Part print with two shaded views. Sizes in mm from the minimum x, y, z corner. Give positions to 0.01 mm unless a question says otherwise; leave off trailing zeros. Loops run counter-clockwise (first coordinate to the right, second up) from the corner with the lowest first, then second, coordinate; pieces in that order, holes last. Notation, with made-up numbers: M -23,70 L 12,70 A37 cw 12,109 Z; hole C 33,-2 d3. An arc over 180 degrees is marked long. Answer as a JSON object with one key per item and string values. Group by question number.
1. Mould opens along Z. For the marked faces 1 and 2 say: released by +Z, released by -Z, zero draft, split by the parting line, or undercut.
2. Slice it at C-C (z = 2.5). List the corners of the cut face in (x, y).
3. Drop flat-ended pins along their axis: pin 1 Ø1 at (y, z) = (42, 21.5) entering from -X; pin 2 Ø6 at (x, z) = (11, 7.5) entering from -Y; pin 3 Ø10 at (x, y) = (18, 37) entering from -Z. Give the stop position or say it passes through.
4. Slice it at A-A (z = 12.5). List the corners of the cut face in (x, y) (1 decimal).
5. Slice it at D-D (y = 24.13). List the corners of the cut face in (x, z).
6. Drill centre lines: line 1 along Z through (x, y) = (24.13, 44.25); line 2 along Y through (x, z) = (27, 20.5) (1 decimal); line 3 along Y through (x, z) = (21, 6). Where is each one in solid material? Low to high. Write a range as [from, to].
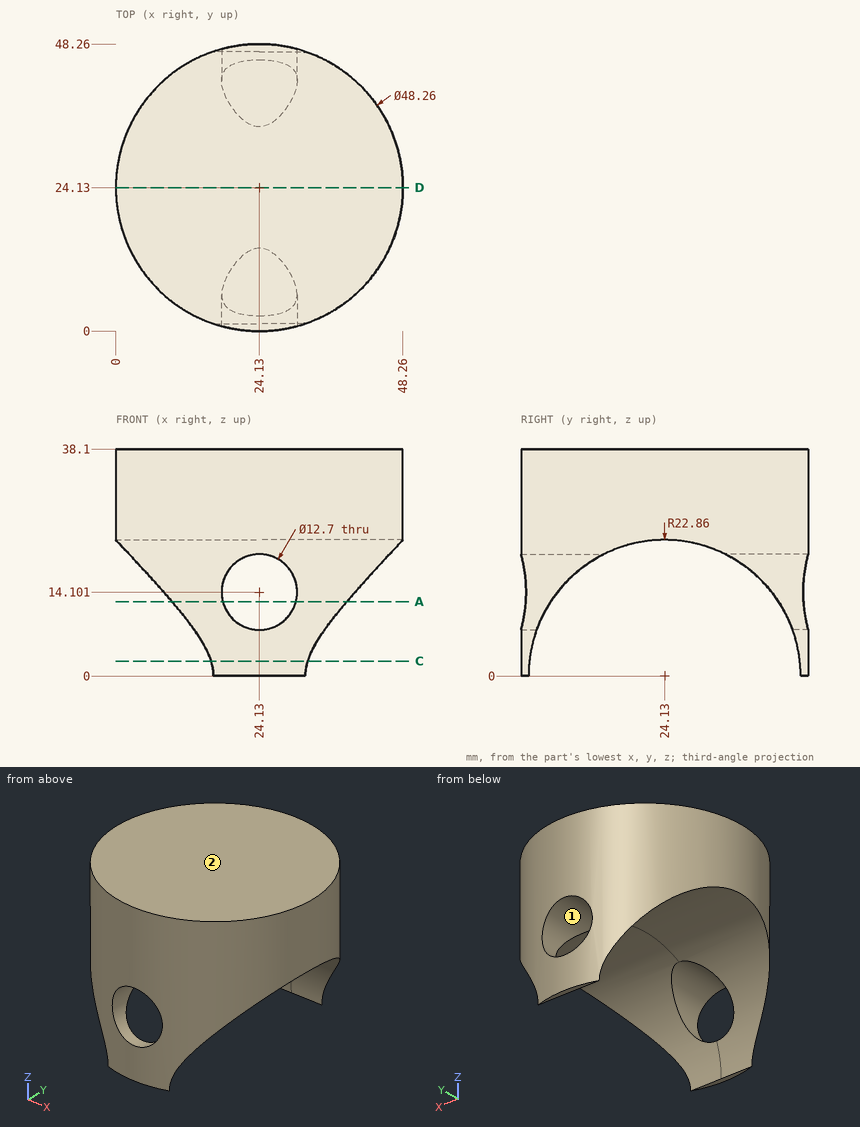
Established:
{
 "1": {"face 1": "undercut", "face 2": "released by +Z"},
 "2": {"outline": "M 16.01,1.41 A24.13 ccw 32.25,1.41 Z; M 16.01,46.85 L 32.25,46.85 A24.13 ccw Z"},
 "3": {"pin 1": "stops at x = 7.38", "pin 2": "stops at y = 2.23", "pin 3": "stops at z = 14.26"},
 "4": {"outline": "M 9.4,5 A24.1 ccw 18,0.8 L 18,5 Z; M 9.4,43.3 L 18,43.3 L 18,47.5 A24.1 ccw Z; M 30.3,0.8 A24.1 ccw 38.8,5 L 30.3,5 Z; M 30.3,43.3 L 38.8,43.3 A24.1 ccw 30.3,47.5 Z"},
 "5": {"outline": "M 0,22.86 L 48.26,22.86 L 48.26,38.1 L 0,38.1 Z"},
 "6": {"line 1": "z = [20.45, 38.1]", "line 2": "y = [0.2, 14], [34.2, 48.1]", "line 3": "y = [0.2, 2.07], [46.19, 48.06]"}
}
